```python
from build123d import *

# Parameters (mm, degrees)
SKETCH_W      = 90
SKETCH_H      = 40
SKETCH_W_2    = 20.4
SKETCH_H_2    = 20.4
PAD_DEPTH     = 10
PAD001_DEPTH  = 10
SKETCH002_R   = 2.75
HOLE_DEPTH    = 40.001
SKETCH003_R   = 2.75
HOLE001_DEPTH = 36.001
SKETCH004_W   = 80
SKETCH004_H   = 5
PAD002_DEPTH  = 10
SKETCH005_R   = 5
SKETCH005_R_2 = 2.75
PAD003_DEPTH  = 1
CHAMFER_SIZE  = 0.99


with BuildPart() as part:
    # Sketch → Pad (new body)
    with BuildSketch(Plane.XY):
        with Locations((45, -20)):
            Rectangle(SKETCH_W, SKETCH_H)
        with Locations((15.2, -15.2)):
            Rectangle(SKETCH_W_2, SKETCH_H_2, mode=Mode.SUBTRACT)
        with Locations((70.2, -15.2)):
            Rectangle(SKETCH_W_2, SKETCH_H_2, mode=Mode.SUBTRACT)
    extrude(amount=PAD_DEPTH)

    # Sketch001 (on Face2 of Pad) → Pad001 (join)
    with BuildSketch(Plane.YZ.offset(90)):
        Polygon((0, 36), (-5, 36), (-5, 23), (-25.4, 23), (-25.4, 36), (-40, 36), (-40, 0), (0, 0), align=None)
    extrude(amount=-PAD001_DEPTH)

    # Sketch002 → Hole (cut, through all)
    with BuildSketch(Plane.XZ):
        with Locations((85, 31)):
            Circle(SKETCH002_R)
    extrude(amount=HOLE_DEPTH, mode=Mode.SUBTRACT)

    # Sketch003 → Hole001 (cut, through all)
    with BuildSketch(Plane.XY):
        with Locations((10.25, -35)):
            Circle(SKETCH003_R)
        with Locations((65.25, -35)):
            Circle(SKETCH003_R)
    extrude(amount=HOLE001_DEPTH, mode=Mode.SUBTRACT)

    # Sketch004 (on Face1 of Hole001) → Pad002 (join)
    with BuildSketch(Plane(origin=(0, 0, 0), x_dir=(-1, 0, 0), z_dir=(0, 1, 0))):
        with Locations((-40, 12.5)):
            Rectangle(SKETCH004_W, SKETCH004_H)
    extrude(amount=-PAD002_DEPTH)

    # Sketch005 → Pad003 (join)
    with BuildSketch(Plane.XY.offset(10)):
        with Locations((10.25, -35)):
            Circle(SKETCH005_R)
        with Locations((10.25, -35)):
            Circle(SKETCH005_R_2, mode=Mode.SUBTRACT)
        with Locations((65.25, -35)):
            Circle(SKETCH005_R)
        with Locations((65.25, -35)):
            Circle(SKETCH005_R_2, mode=Mode.SUBTRACT)
    extrude(amount=PAD003_DEPTH)

    # Chamfer
    chamfer_edges = [part.edges().sort_by_distance(p)[0] for p in [
        (5.25, -35, 11),
        (60.25, -35, 11),
    ]]
    chamfer(chamfer_edges, length=CHAMFER_SIZE)


solid = part.part
```
Verification items for the finished model (mm, model axes). A direction names the side the tool comes from. Coordinates: 2 decimals unless noted, no trailing zeros. Loops run counter-clockwise (first coordinate to the right, second up) from the corner with the lowest first, then second, coordinate; pieces in that order, holes last. Notation, with made-up numbers: (7.5, 20.25) -> (39.5, 20.25) arc R23 cw to (39.5, 28.25) -> close; hole circle Ø5 at (89, -7.5). An arc over 180 degrees is marked (long way). Answer in a Markdown table with one row per item. Add a question column.
1. Section check B-B, the plane z = 31. Enter the section's corners in (x, y), then the cut area to 3 significant figures.
2. Section check D-D, the plane x = 72. Enter the section's corners in (y, z).
3. Section check A-A, the plane y = -12. Enter the section's corners in (x, z).
4. Section check C-C, the plane y = -35. Give the number of separate pieces and of enclosed holes in the cut face, then the cut area to 3 significant figures.
5. Material ranges on probe 1 along Y at (x, z) = (65.25, 3); probe 2 along Y at (x, z) = (61.5, 9); probe 3 along X at (y, z) = (-30, 31), recorded low to high. Write a range as [from, to].
6. Access from +Z, -Z, +X, -X, +Y, -Y to the whole of each face (thin tool, end or side, straight path). Record for faces 4 (the face through (85, -33, 36)), 5 (the face through (85, -15, 23)), 6 (the face through (60, -15, 5)).
7. Depth check by flat-ended pin: P1, Ø4, axis at x = 37, y = -33.5, coming from the +Z side; P2, Ø3.5, axis at x = 85, z = 31, coming from the +Y side; P3, Ø4, axis at x = 22.5, z = 13, coming from the -Y side; P4, Ø2.5, axis at x = 70, y = -7.5, coming from the -Z side. Enter the tip coordinate at first touch or a pass-through.
8. Draft check along Y on faces 1 (the face through (85, -25.4, 28)), 2 (the face through (68, -34, 11)), 3 (the face through (52, -40, 9)). Enter one of: +Y half, -Y half, draft (parallel to the pull), parting line (faces both ways), or undercut.
Derived:
| question | item | result |
|---|---|---|
| 1 | outline | (80, -40) -> (82.25, -40) -> (82.25, -25.4) -> (80, -25.4) -> close; (80, -5) -> (82.25, -5) -> (82.25, 0) -> (80, 0) -> close; (87.75, -40) -> (90, -40) -> (90, -25.4) -> (87.75, -25.4) -> close; (87.75, -5) -> (90, -5) -> (90, 0) -> (87.75, 0) -> close |
| 1 | area | 88.2 mm² |
| 2 | outline | (-40, 0) -> (-25.4, 0) -> (-25.4, 10) -> (-40, 10) -> close; (-10, 10) -> (-5, 10) -> (-5, 0) -> (0, 0) -> (0, 15) -> (-10, 15) -> close |
| 3 | outline | (0, 0) -> (5, 0) -> (5, 10) -> (0, 10) -> close; (25.4, 0) -> (60, 0) -> (60, 10) -> (25.4, 10) -> close; (80, 0) -> (90, 0) -> (90, 23) -> (80, 23) -> close |
| 4 | separate pieces | 3 |
| 4 | enclosed holes | 1 |
| 4 | area | 1,030 mm² |
| 5 | probe 1 | y = [-40, -37.75], [-32.25, -25.4], [-5, 0] |
| 5 | probe 2 | y = [-40, -25.4], [-5, 0] |
| 5 | probe 3 | x = [80, 82.25], [87.75, 90] |
| 6 | face 4 | +Z, +X, -X, +Y, -Y |
| 6 | face 5 | +Z, +X, -X |
| 6 | face 6 | -Z |
| 7 | P1 | stops at z = 10 |
| 7 | P2 | passes through |
| 7 | P3 | stops at y = -10 |
| 7 | P4 | stops at z = 10 |
| 8 | face 1 | undercut |
| 8 | face 2 | draft |
| 8 | face 3 | -Y half |
